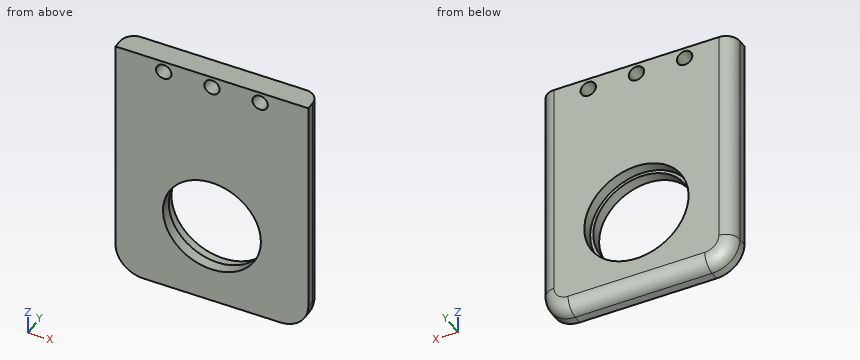
from build123d import *

# Parameters (mm, degrees)
SKETCH1_W           = 68.9
SKETCH1_H           = 90
SKETCH1_R           = 18.63
SKETCH1_R_2         = 2.75
BOSS_EXTRUDE1_DEPTH = 8
FILLET1_R           = 10
FILLET2_R           = 5
SKETCH2_R           = 18.63
SKETCH2_R_2         = 17.5
BOSS_EXTRUDE2_DEPTH = 4


with BuildPart() as part:
    # Sketch1 → Boss-Extrude1 (new body)
    with BuildSketch(Plane(origin=(0, 0, 0), x_dir=(1, 0, 0), z_dir=(0, 1, 0))):
        with Locations((0.722348924, 5)):
            Rectangle(SKETCH1_W, SKETCH1_H)
        with Locations(Location((0.722348924, 20, 0), (0, 0, 270))):
            Circle(SKETCH1_R, mode=Mode.SUBTRACT)
        with Locations(Location((0.722348924, -36, 0), (0, 0, 270))):
            Circle(SKETCH1_R_2, mode=Mode.SUBTRACT)
        with Locations(Location((-16.502651076, -36, 0), (0, 0, 270))):
            Circle(SKETCH1_R_2, mode=Mode.SUBTRACT)
        with Locations(Location((17.947348924, -36, 0), (0, 0, 270))):
            Circle(SKETCH1_R_2, mode=Mode.SUBTRACT)
    extrude(amount=BOSS_EXTRUDE1_DEPTH)

    # Fillet1
    fillet1_edges = [part.edges().sort_by_distance(p)[0] for p in [
        (-33.727651076, 4, -50),
        (35.172348924, 4, -50),
    ]]
    fillet(fillet1_edges, radius=FILLET1_R)

    # Fillet2
    fillet2_edges = [part.edges().sort_by_distance(p)[0] for p in [
        (35.172348924, 8, 0),
        (0.722348924, 8, -50),
        (-33.727651076, 8, 0),
        (-30.798718888, 8, -47.071067812),
        (32.243416735, 8, -47.071067812),
    ]]
    fillet(fillet2_edges, radius=FILLET2_R)

    # Sketch2 → Boss-Extrude2 (add)
    with BuildSketch(Plane.XZ):
        with Locations(Location((0.722348924, -20, 0), (0, 0, 270))):
            Circle(SKETCH2_R)
        with Locations(Location((0.722348924, -20, 0), (0, 0, 270))):
            Circle(SKETCH2_R_2, mode=Mode.SUBTRACT)
    extrude(amount=-BOSS_EXTRUDE2_DEPTH)


solid = part.part
Could you check a few things on this model? Use its own coordinates, in mm. Coordinates: 2 decimals unless noted, no trailing zeros. Order: outer loops, then holes, each group sorted by start corner. A loop starts at its lowest first (then second) coordinate and runs counter-clockwise, first axis right, second up.
Q1. Please list where these lines run through material, in increasing order: L1, parallel to X at y = 3.25, z = 36; L2, parallel to Z at x = -14, y = 6; L3, parallel to Z at x = -1.5, y = 2.5.
Q2. Will this pin go through, and if not, where does the flat tip stop? pin 1 (4 mm diameter, centred on y = 5.5, z = -8.5, fed in from +X).
Q3. Suppose I cut it at B-B on z = -20. Please give me the cut outline in (x, y), and give its area (3 significant figures).
Q4. Suppose I cut it at C-C on x = -7.5. Please give me the cut outline in (y, z).
Q5. Suppose I cut it at D-D on z = 22. Please give me the cut outline in (x, y), and give its area (3 significant figures).
Q6. Suppose I cut it at A-A on z = 36. Please give me the cut outline in (x, y).
Answer:
1. L1: x = -33.72 to -19.25, -13.75 to -2.03, 3.47 to 15.2, 20.7 to 35.17
1. L2: z = -49 to -31.42, -8.58 to 34.86, 37.14 to 40
1. L3: z = -50 to -37.36, -2.64 to 34.38, 37.62 to 40
2. pin 1: stops at x = 35.15
3. outline: (-33.73, 0) - (-16.78, 0) - (-16.78, 4) - (-17.91, 4) - (-17.91, 8) - (-28.73, 8) arc R5 ccw to (-33.73, 3) - close; (18.22, 0) - (35.17, 0) - (35.17, 3) arc R5 ccw to (30.17, 8) - (19.35, 8) - (19.35, 4) - (18.22, 4) - close
3. area: 251 mm2
4. outline: (0, -50) - (3, -50) arc R5 ccw to (8, -45) - (8, -36.72) - (4, -36.72) - (4, -35.45) - (0, -35.45) - close; (0, -4.55) - (4, -4.55) - (4, -3.28) - (8, -3.28) - (8, 40) - (0, 40) - close
5. outline: (-33.73, 0) - (35.17, 0) - (35.17, 3) arc R5 ccw to (30.17, 8) - (-28.73, 8) arc R5 ccw to (-33.73, 3) - close
5. area: 540 mm2
6. outline: (-33.73, 0) - (-19.25, 0) - (-19.25, 8) - (-28.73, 8) arc R5 ccw to (-33.73, 3) - close; (-13.75, 0) - (-2.03, 0) - (-2.03, 8) - (-13.75, 8) - close; (3.47, 0) - (15.2, 0) - (15.2, 8) - (3.47, 8) - close; (20.7, 0) - (35.17, 0) - (35.17, 3) arc R5 ccw to (30.17, 8) - (20.7, 8) - close
